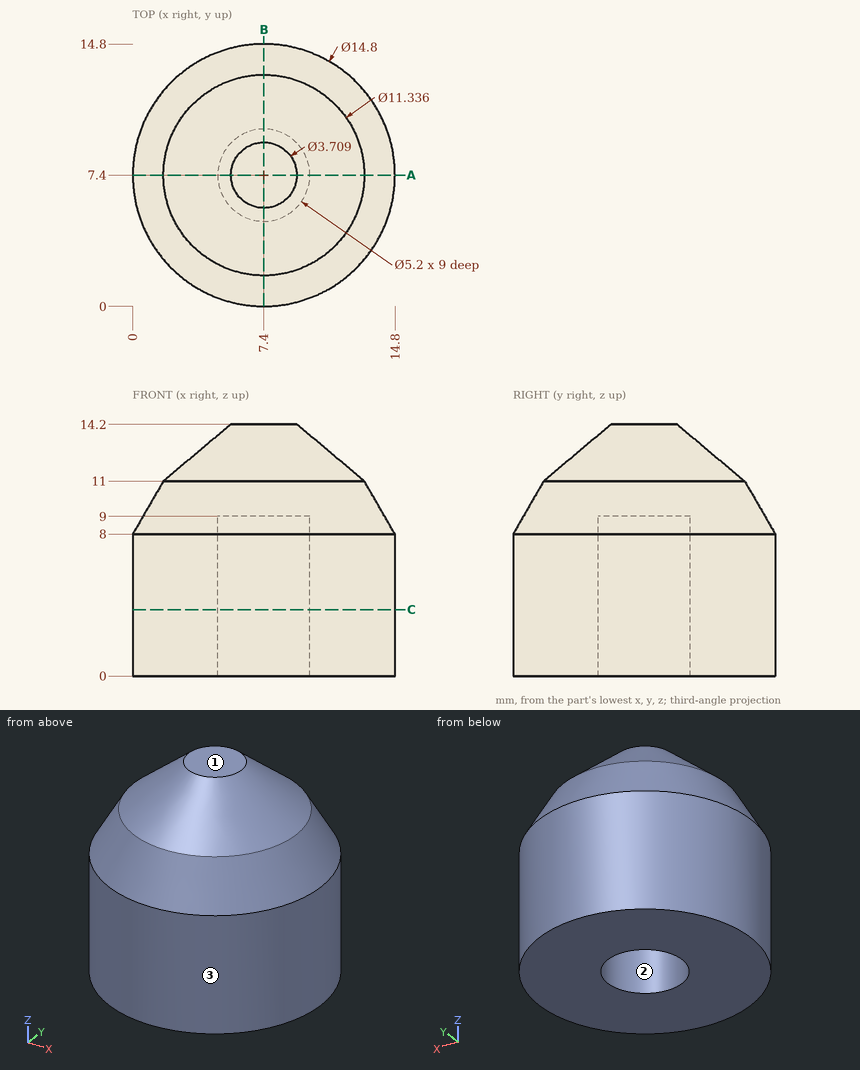
Print and shaded views of the part. All mm, measured from the part's lowest x, y and z. Round coordinates to 2 decimals unless told otherwise and drop trailing zeros. Write each loop counter-clockwise with the first axis right and the second up, starting at its lowest first coordinate (ties: lowest second). Pieces come first, ordered by that corner, then holes.
Item 1: Two-plate mould, pull along X, no slides. Class the marked faces 1, 2 and 3: +X half, -X half, draft (parallel to the pull), parting line (faces both ways), or undercut.
Results:
face 1: draft
face 2: undercut
face 3: parting line
Item 2: Cut at A-A, the plane y = 7.4. Give the cut face in (x, z).
Results:
outline: (0, 0) - (4.8, 0) - (4.8, 9) - (10, 9) - (10, 0) - (14.8, 0) - (14.8, 8) - (13.07, 11) - (9.25, 14.2) - (5.55, 14.2) - (1.73, 11) - (0, 8) - close
Item 3: Probe L1, parallel to Y at x = 7.4, z = 7; L2, parallel to Z at x = 9, y = 8; L3, parallel to Y at x = 6.5, z = 6.25 (1 decimal). List the from-to ranges inside material, lowest first.
Results:
L1: y = 0 to 4.8, 10 to 14.8
L2: z = 9 to 14.2
L3: y = 0.1 to 5, 9.8 to 14.7
Item 4: Drop flat-ended pins along their axis: pin 1 Ø3 at (x, z) = (4, 12.5) entering from -Y (1 decimal); pin 2 Ø2 at (x, y) = (12.5, 7.5) entering from +Z (1 decimal); pin 3 Ø2 at (x, y) = (2, 9) entering from +Z. Give the stop position or say it passes through.
Results:
pin 1: stops at y = 2.6
pin 2: stops at z = 12.3
pin 3: stops at z = 11.87
Item 5: Cut at C-C, the plane z = 3.75. Give the cut face in (x, y), plus the area to 3 significant figures.
Results:
outline: circle Ø14.8 at (7.4, 7.4); hole circle Ø5.2 at (7.4, 7.4)
area: 151 mm2
